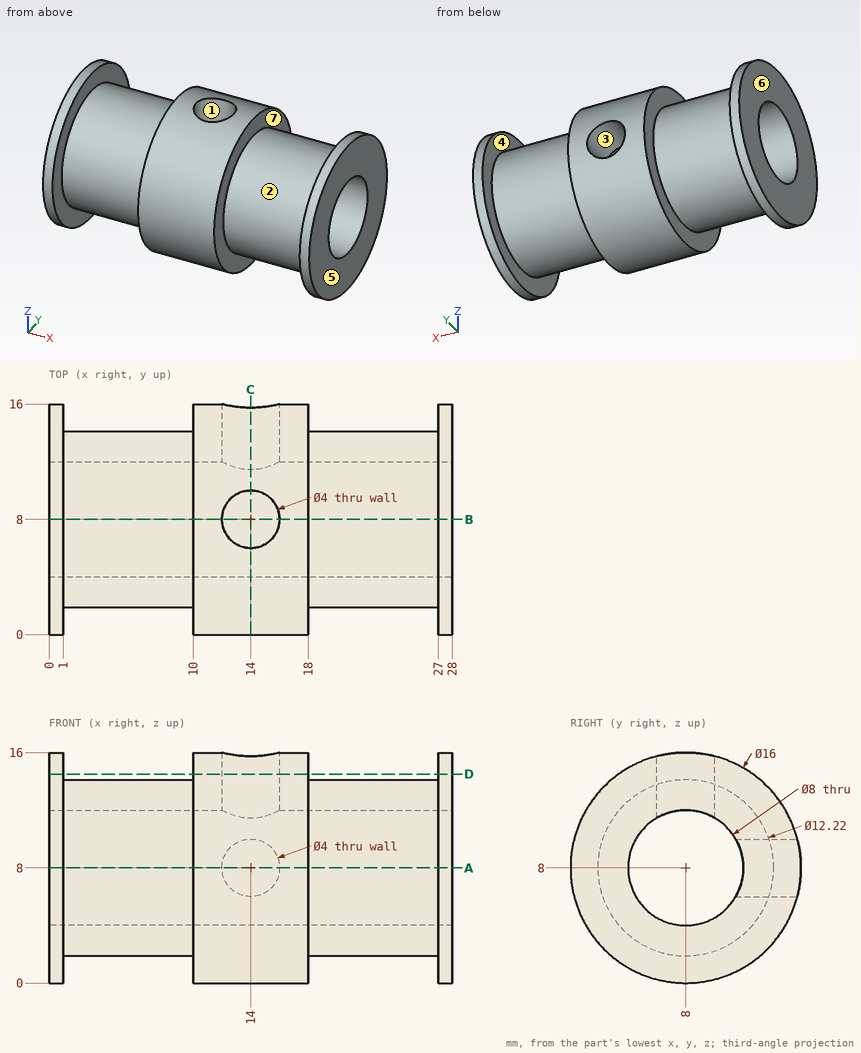
Job drawing, mm, ordinate dimensions from the low corner. One solid piece. A direction names the side the tool comes from. Give positions to 0.01 mm unless a question says otherwise; leave off trailing zeros. Order: outer loops, then holes, each group sorted by start corner. A loop starts at its lowest first (then second) coordinate and runs counter-clockwise, first axis right, second up. Notation, with made-up numbers: (-19, -14.5) -> (7, -14.5) arc R27 cw to (7, 7.5) -> close; hole circle Ø1 at (51, 6). An arc over 180 degrees is marked (long way). Return JSON: item names as keys, results as strings.
Q1. Saw through at D-D (z = 14.5). Write the cut outline in (x, y), then the cut area to 3 significant figures.
Working result:
{"outline": "(0, 3.34) -> (1, 3.34) -> (1, 12.66) -> (0, 12.66) -> close; (10, 3.34) -> (18, 3.34) -> (18, 12.66) -> (10, 12.66) -> close; (27, 3.34) -> (28, 3.34) -> (28, 12.66) -> (27, 12.66) -> close; hole circle Ø4 at (14, 8)", "area": "80.7 mm²"}
Q2. Saw through at C-C (x = 14). Write the cut outline in (y, z).
Working result:
{"outline": "(6, 11.46) -> (6, 15.75) arc R8 ccw (long way) to (15.75, 6) -> (11.46, 6) arc R4 cw (long way) to start; (10, 11.46) arc R4 cw to (11.46, 10) -> (15.75, 10) arc R8 ccw to (10, 15.75) -> close"}
Q3. Which spindle directions (+Z, -Z, +X, -X, +Y, -Y) get a long thin tool onto all of the face, cutting with end or side? Do the marked faces 1, 2 and 3. Say none if no direction does.
Working result:
{"face 1": "+Z", "face 2": "none", "face 3": "+Y"}
Q4. Flat gauge pins, fed straight in: pin 1 (2.5 mm diameter, centred on x = 14, z = 8, fed in from +Y); pin 2 (3 mm diameter, centred on x = 18, z = 3, fed in from -Y); pin 3 (2 mm diameter, centred on x = 21, z = 2.5, fed in from -Y). Where does each tip first touch, or does it go through?
Working result:
{"pin 1": "y = 4.2", "pin 2": "y = 0.81", "pin 3": "y = 3.87"}
Q5. Saw through at A-A (z = 8). Write the cut outline in (x, y), then the cut area to 3 significant figures.
Working result:
{"outline": "(0, 0) -> (1, 0) -> (1, 1.89) -> (10, 1.89) -> (10, 0) -> (18, 0) -> (18, 1.89) -> (27, 1.89) -> (27, 0) -> (28, 0) -> (28, 4) -> (0, 4) -> close; (0, 12) -> (12, 12) -> (12, 16) -> (10, 16) -> (10, 14.11) -> (1, 14.11) -> (1, 16) -> (0, 16) -> close; (16, 12) -> (28, 12) -> (28, 16) -> (27, 16) -> (27, 14.11) -> (18, 14.11) -> (18, 16) -> (16, 16) -> close", "area": "140 mm²"}
Q6. Mould opens along X. For the marked faces 4, 5, 6 and 7 say: pulls with the +X half, pulls with the -X half, needs draft (parallel to the pull), parting line crosses it, or undercut.
Working result:
{"face 4": "undercut", "face 5": "pulls with the +X half", "face 6": "pulls with the -X half", "face 7": "undercut"}
Q7. Drill centre lines: line 1 (X direction, y = 3.5, z = 2.5); line 2 (Y direction, x = 2.25, z = 7.5); line 3 (Z direction, x = 14, y = 13.65). Where is each one in solid material? Low to high.
Working result:
{"line 1": "0 to 1, 10 to 18, 27 to 28", "line 2": "1.91 to 4.03, 11.97 to 14.09", "line 3": "2.34 to 6, 10 to 13.66"}
